Read the model definition and answer for the solid it produces. Units are mm, in the model's axes. Coordinates: 2 decimals unless noted, no trailing zeros. Loops run counter-clockwise (first coordinate to the right, second up) from the corner with the lowest first, then second, coordinate; pieces in that order, holes last.
from build123d import *

# Parameters (mm, degrees)
F0_R     = 0.4
F1_DEPTH = 47


with BuildPart() as f1:
    # F0 (on Front) → F1 (new body)
    with BuildSketch(Plane.XZ):
        with BuildLine():
            Line((-0.7, 0.55), (-0.7, -0.55))
            ThreePointArc((-0.7, -0.55), (0, -1.25), (0.7, -0.55))
            Line((0.7, -0.55), (0.7, 0.55))
            ThreePointArc((0.7, 0.55), (0, 1.25), (-0.7, 0.55))
        make_face()
        with Locations((0, -0.55)):
            Circle(F0_R, mode=Mode.SUBTRACT)
        with Locations((0, 0.55)):
            Circle(F0_R, mode=Mode.SUBTRACT)
    extrude(amount=-F1_DEPTH)


solid = f1.part
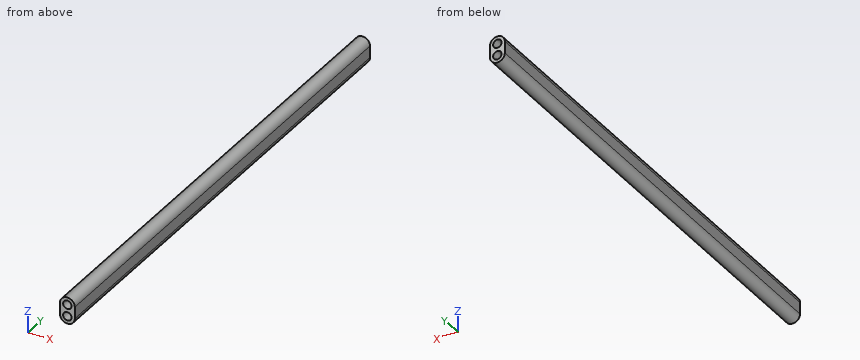
Item 1: A cutting plane is placed at B-B on y = 23. Determine the outline of the cut face in (x, z), then the cut area to 3 significant figures.
Numbers:
outline: (-0.7, -0.55) arc R0.7 ccw to (0.7, -0.55) - (0.7, 0.55) arc R0.7 ccw to (-0.7, 0.55) - close; hole circle Ø0.8 at (0, -0.55); hole circle Ø0.8 at (0, 0.55)
area: 2.07 mm2
Item 2: Find the intervals of material crossed by line 1 along Z through (x, y) = (-0.05, 36.5); line 2 along X through (y, z) = (44, -0.45); line 3 along X through (y, z) = (45, 1.1), in increasing order.
Numbers:
line 1: z = -1.25 to -0.95, -0.15 to 0.15, 0.95 to 1.25
line 2: x = -0.7 to -0.39, 0.39 to 0.7
line 3: x = -0.43 to 0.43
Item 3: A cutting plane is placed at A-A on x = 0.05. Determine the outline of the cut face in (y, z).
Numbers:
outline: (0, -1.25) - (47, -1.25) - (47, -0.95) - (0, -0.95) - close; (0, -0.15) - (47, -0.15) - (47, 0.15) - (0, 0.15) - close; (0, 0.95) - (47, 0.95) - (47, 1.25) - (0, 1.25) - close
